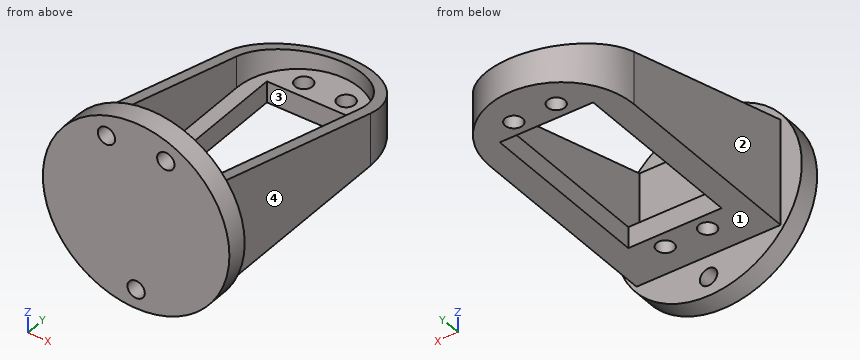
```python
from build123d import *

# Parameters (mm, degrees)
SKETCH1_W           = 22
SKETCH1_H           = 42
SKETCH1_R           = 2.05
BOSS_EXTRUDE1_DEPTH = 5
BOSS_EXTRUDE2_DEPTH = 20
CUT_EXTRUDE1_DEPTH  = 35
SKETCH4_R           = 22
BOSS_EXTRUDE3_DEPTH = 5
SKETCH5_R           = 2.05
CUT_EXTRUDE2_DEPTH  = 5


with BuildPart() as part:
    # Sketch1 → Boss-Extrude1 (new body)
    with BuildSketch(Plane.XY):
        with BuildLine():
            Line((17, -32), (17, 16))
            ThreePointArc((17, 16), (0, 33), (-17, 16))
            Line((-17, 16), (-17, -32))
            Line((-17, -32), (17, -32))
        make_face()
        Rectangle(SKETCH1_W, SKETCH1_H, mode=Mode.SUBTRACT)
        with Locations((-5, -24.75)):
            Circle(SKETCH1_R, mode=Mode.SUBTRACT)
        with Locations((5, -24.75)):
            Circle(SKETCH1_R, mode=Mode.SUBTRACT)
        with Locations((-5, 24.75)):
            Circle(SKETCH1_R, mode=Mode.SUBTRACT)
        with Locations((5, 24.75)):
            Circle(SKETCH1_R, mode=Mode.SUBTRACT)
    extrude(amount=BOSS_EXTRUDE1_DEPTH)

    # Sketch2 → Boss-Extrude2 (add)
    with BuildSketch(Plane.XY.offset(5)):
        with BuildLine():
            Line((17, -32), (17, 16))
            ThreePointArc((17, 16), (0, 33), (-17, 16))
            Line((-17, 16), (-17, -32))
            Line((-17, -32), (17, -32))
        make_face()
        with BuildLine():
            Line((-14.5, 16), (-14.5, -29.5))
            Line((-14.5, -29.5), (14.5, -29.5))
            Line((14.5, -29.5), (14.5, 16))
            ThreePointArc((14.5, 16), (0, 30.5), (-14.5, 16))
        make_face(mode=Mode.SUBTRACT)
    extrude(amount=BOSS_EXTRUDE2_DEPTH)

    # Sketch3 → Cut-Extrude1 (cut, through all)
    with BuildSketch(Plane(origin=(17, 0, 0), x_dir=(0, 0, -1), z_dir=(1, 0, 0))):
        Polygon((-25, -32), (-8, 33), (-25, 33), align=None)
    extrude(amount=-CUT_EXTRUDE1_DEPTH, mode=Mode.SUBTRACT)

    # Sketch4 → Boss-Extrude3 (add)
    with BuildSketch(Plane.XZ.offset(32)):
        with Locations((0, 12.5)):
            Circle(SKETCH4_R)
    extrude(amount=BOSS_EXTRUDE3_DEPTH)

    # Sketch5 → Cut-Extrude2 (cut)
    with BuildSketch(Plane(origin=(0, -32, 0), x_dir=(1, 0, 0), z_dir=(0, 1, 0))):
        with Locations((0, 5)):
            Circle(SKETCH5_R)
        with Locations((-7, -28.5)):
            Circle(SKETCH5_R)
        with Locations((7, -28.5)):
            Circle(SKETCH5_R)
    extrude(amount=-CUT_EXTRUDE2_DEPTH, mode=Mode.SUBTRACT)


solid = part.part
```
Build history of the part. All positions in model axes, mm. Face numbers are marked on the shaded views. A direction names the side the tool comes from. Give positions to 0.01 mm unless a question says otherwise; leave off trailing zeros. Order: outer loops, then holes, each group sorted by start corner. A loop starts at its lowest first (then second) coordinate and runs counter-clockwise, first axis right, second up. Notation, with made-up numbers: M 58,60 L 65,60 A7 ccw 65,66 Z; hole C 56.5,-19.5 d4. An arc over 180 degrees is marked long. Return JSON: item names as keys, results as strings.
Q1. Band-saw the part on C-C (x = 10). Give the cut face in (y, z).
Answer list:
{"outline": "M -37,-7.1 L -32,-7.1 L -32,0 L -21,0 L -21,5 L -29.5,5 L -29.5,24.35 L -32,25 L -32,32.1 L -37,32.1 Z; M 21,0 L 29.75,0 L 29.75,8.85 L 26.5,9.7 L 26.5,5 L 21,5 Z"}
Q2. Band-saw the part on D-D (z = 28.5). Give the cut face in (x, y), then the cut area to 3 significant figures.
Answer list:
{"outline": "M -15.1,-37 L -9.05,-37 L -9.05,-32 L -15.1,-32 Z; M -4.95,-37 L 4.95,-37 L 4.95,-32 L -4.95,-32 Z; M 9.05,-37 L 15.1,-37 L 15.1,-32 L 9.05,-32 Z", "area": "110 mm^2"}
Q3. Band-saw the part on B-B (y = -3.5). Give the cut face in (x, z), then the cut area to 3 significant figures.
Answer list:
{"outline": "M -17,0 L -11,0 L -11,5 L -14.5,5 L -14.5,17.55 L -17,17.55 Z; M 11,0 L 17,0 L 17,17.55 L 14.5,17.55 L 14.5,5 L 11,5 Z", "area": "123 mm^2"}
Q4. Wall check: probe 1 along Y at (x, z) = (5, 1); probe 2 along X at (y, z) = (-35, 28); probe 3 along X at (y, z) = (-20, 2.5). Give the ranges that are in metal, low to high. Write a range as from..to.
Answer list:
{"probe 1": "y = -37..-26.8, -22.7..-21, 21..22.7, 26.8..32.25", "probe 2": "x = -15.61..-8.99, -5.01..5.01, 8.99..15.61", "probe 3": "x = -17..-11, 11..17"}
Q5. Band-saw the part on A-A (z = -5). Give the cut face in (x, y).
Answer list:
{"outline": "M -13.33,-37 L -2.05,-37 L -2.05,-32 L -13.33,-32 Z; M 2.05,-37 L 13.33,-37 L 13.33,-32 L 2.05,-32 Z"}
Q6. 3-axis set-ups, long thin cutter, end or side, ignore diameter. For the marked faces 1, 2, 3 and 4: which of +Z, -Z, +X, -X, +Y, -Y reach the whole face in a straight line?
Answer list:
{"face 1": "-Z, +X, -X, +Y", "face 2": "+Z, -Z, -X, +Y", "face 3": "+Z, -Z", "face 4": "+Z, -Z, +X, +Y"}
Q7. Flat gauge pins, fed straight in: pin 1 (21.5 mm diameter, centred on y = -14, z = 14, fed in from -X); pin 2 (4.5 mm diameter, centred on x = 0, z = -5, fed in from +Y); pin 3 (23 mm diameter, centred on x = 1, y = -11, fed in from +Z); pin 4 (13 mm diameter, centred on x = 4.5, z = 2, fed in from +Y). Where does each tip first touch, or does it go through?
Answer list:
{"pin 1": "stops at x = -17", "pin 2": "stops at y = -32", "pin 3": "stops at z = 5", "pin 4": "stops at y = 33"}
